Autodesk Inventor part; units mm, degrees
ref_plane "YZ Plane" through (0, 0, 0) normal (1, 0, 0) x (0, 1, 0)
ref_plane "XZ Plane" through (0, 0, 0) normal (0, 1, 0) x (-1, 0, 0)
ref_plane "XY Plane" through (0, 0, 0) normal (0, 0, 1) x (1, 0, 0)
sketch "Sketch1" plane through (0, 0, 0) normal (0, 0, 1) x (1, 0, 0)
  line L0 (-6.5, -6.5) -> (6.5, -6.5)
  line L1 (6.5, -6.5) -> (6.5, 6.5)
  line L2 (6.5, 6.5) -> (-6.5, 6.5)
  line L3 (-6.5, 6.5) -> (-6.5, -6.5)
  line L4 (-6.5, -6.5) -> (6.5, 6.5) construction
  line L5 (6.5, -6.5) -> (-6.5, 6.5) construction
  line L6 (-5.5, -5.5) -> (5.5, -5.5)
  line L7 (5.5, -5.5) -> (5.5, 5.5)
  line L8 (5.5, 5.5) -> (-5.5, 5.5)
  line L9 (-5.5, 5.5) -> (-5.5, -5.5)
  line L10 (-5.5, -5.5) -> (5.5, 5.5) construction
  line L11 (5.5, -5.5) -> (-5.5, 5.5) construction
  line L12 (5.5, 5.5) -> (6.5, 5.5)
  line L13 (6.5, 5.5) -> (6.5, 4.5)
  line L14 (6.5, 4.5) -> (5.5, 4.5)
  line L15 (5.5, 4.5) -> (5.5, 5.5)
  line L16 (5.5, -5.5) -> (6.5, -5.5)
  line L17 (6.5, -5.5) -> (6.5, -4.5)
  line L18 (6.5, -4.5) -> (5.5, -4.5)
  line L19 (5.5, -4.5) -> (5.5, -5.5)
  point P0 (0, 0)
  point P1 (5.5, -4.5)
  point P2 (5.5, 4.5)
  dimension "d0" = 13
  dimension "d1" = 13
  dimension "d2" = 11
  dimension "d3" = 11
  dimension "d4" = 1
  dimension "d5" = 1
extrude "Extrusion1" add sketch "Sketch1" along normal blind 4
extrude "Extrusion2" cut sketch "Sketch1" along normal blind 2 contours L18 L7 L14 L1 | L6 L9 L8 L7
sketch "Sketch2" plane through (0, 0, 2) normal (0, 0, -1) x (-1, 0, 0)
  line L0 (-6.5, -6.5) -> (-6.5, 6.5)
  line L1 (-5.5, -4.5) -> (-6.5, -4.5)
  line L2 (-6.5, 4.5) -> (-5.5, 4.5)
  line L3 (-5.5, 4.5) -> (-5.5, -4.5)
  line L4 (-5.5, -4.5) -> (-6.5, -4.5)
  line L5 (-6.5, -4.5) -> (-6.5, 4.5)
  line L6 (-6.5, 4.5) -> (-5.5, 4.5)
  line L7 (5.5, 5.5) -> (5.5, -5.5)
  line L8 (-5.5, 4.5) -> (5.5, 4.5)
  line L9 (5.5, 4.5) -> (5.5, -4.5)
  line L10 (5.5, -4.5) -> (-5.5, -4.5)
  line L11 (-5.5, -4.5) -> (-5.5, 4.5)
  point P0 (0, 0)
  dimension "d18" = 0
extrude "Extrusion3" cut sketch "Sketch2" against normal blind 1
sketch "Sketch3" plane through (0, 0, 0) normal (0, 0, -1) x (-1, 0, 0)
  line L0 (6.5, 6.5) -> (6.5, -6.5)
  line L1 (5.5, 5.5) -> (5.5, -5.5)
  line L2 (6.5, 5.5) -> (5.5, 5.5)
  line L3 (5.5, 5.5) -> (5.5, -5.5)
  line L4 (5.5, -5.5) -> (6.5, -5.5)
  line L5 (6.5, -5.5) -> (6.5, 5.5)
  line L6 (-5.5, 5.5) -> (5.5, 5.5)
  point P0 (0, 0)
  point P1 (5.5, 5.5)
  dimension "d15" = 0
extrude "Extrusion4" cut sketch "Sketch3" against normal blind 2
properties part number "Optical module_lid_2"
The listing builds one solid part. Answer for the finished solid, in the listing's coordinates (mm). A direction names the side the tool comes from. Coordinates: 2 decimals unless noted, no trailing zeros. Write each loop counter-clockwise with the first axis right and the second up, starting at its lowest first coordinate (ties: lowest second). Pieces come first, ordered by that corner, then holes. Notation, with made-up numbers: M -27,12 L 6,12 A28 cw 6,40 Z; hole C 21.25,73 d1. An arc over 180 degrees is marked long. Put each result on its own line as item: value. Start each with the question number.
1. Consider line 1 (Y direction, x = 4, z = 0.7); line 2 (Y direction, x = -4, z = 2.55); line 3 (Z direction, x = -5, y = -0.25). Determine where each line is inside the solid, lowest interval first. Write a range as from..to.
2. A cutting plane is placed at D-D on y = -5. Write down the section's boundary in (x, z), then the cut area to 3 significant figures.
3. Flat-ended cylindrical pins translate along their axes: P1, Ø0.8, axis at y = -5, z = 0.5, coming from the -X side; P2, Ø3.5, axis at x = -0.5, y = 1, coming from the -Z side; P3, Ø2, axis at x = -1, y = -4, coming from the -Z side. Find the tip coordinate at first contact, or state that the pin passes through.
4. A cutting plane is placed at B-B on x = 2. Write down the section's boundary in (y, z), then the cut area to 3 significant figures.
5. A cutting plane is placed at C-C on y = 0.5. Write down the section's boundary in (x, z).
6. Which of the six approach directions +Z, -Z, +X, -X, +Y, -Y give full straight-line access (tool end or side, diameter ignored) to faces 1 (the flat face through (1.9, -4.5, 2.5)), 2 (the flat face through (5.5, 5, 1)), 3 (the flat face through (0, 0, 4))?
7. A cutting plane is placed at A-A on z = 0.85. Write down the section's boundary in (x, y), then the cut area to 3 significant figures.
8. For a pull along Y with two mould halves and no side action, classify faces 4 (the flat face through (-5.5, 0.1, 2.5)), 5 (the flat face through (0, 6.5, 2)), 6 (the flat face through (6.5, -0.1, 3.3)) as pulls with the +Y half, pulls with the -Y half, needs draft (parallel to the pull), parting line crosses it, or undercut.
Resolved:
1. line 1: y = -6.5..-5.5, 5.5..6.5
1. line 2: y = -6.5..-4.5, 4.5..6.5
1. line 3: z = 3..4
2. outline: M -6.5,2 L 5.5,2 L 5.5,0 L 6.5,0 L 6.5,4 L -6.5,4 Z
2. area: 28.0 mm2
3. P1: stops at x = 5.5
3. P2: stops at z = 3
3. P3: stops at z = 2
4. outline: M -6.5,0 L -5.5,0 L -5.5,2 L -4.5,2 L -4.5,3 L 4.5,3 L 4.5,2 L 5.5,2 L 5.5,0 L 6.5,0 L 6.5,4 L -6.5,4 Z
4. area: 21.0 mm2
5. outline: M -6.5,2 L -5.5,2 L -5.5,3 L 6.5,3 L 6.5,4 L -6.5,4 Z
6. face 1: -Z, +X
6. face 2: -Z, -X
6. face 3: +Z, +X, -X, +Y, -Y
7. outline: M -6.5,-6.5 L 6.5,-6.5 L 6.5,-4.5 L 5.5,-4.5 L 5.5,-5.5 L -6.5,-5.5 Z; M -6.5,5.5 L 5.5,5.5 L 5.5,4.5 L 6.5,4.5 L 6.5,6.5 L -6.5,6.5 Z
7. area: 28.0 mm2
8. face 4: undercut
8. face 5: pulls with the +Y half
8. face 6: needs draft
